from build123d import *

# Parameters (mm, degrees)
BOSS_EXTRUDE1_DEPTH      = 10
BOSS_EXTRUDE1_DEPTH_BACK = 10
SKETCH2_W                = 17.5
SKETCH2_H                = 24
SKETCH3_W                = 9.984775587
SKETCH3_H                = 3
SKETCH3_W_2              = 10
CUT_EXTRUDE1_DEPTH       = 10


with BuildPart() as part:
    # Sketch2 → Boss-Extrude1 (new, two sides: drawn at the far end of the back side and taken through both)
    with BuildSketch(Plane.XY.offset(-BOSS_EXTRUDE1_DEPTH_BACK)):
        with Locations((8.75, -33)):
            Rectangle(SKETCH2_W, SKETCH2_H)
        with Locations((-8.75, -33)):
            Rectangle(SKETCH2_W, SKETCH2_H)
        Polygon((28.106601718, -45), (17.5, -45), (17.5, -21), (24.571067812, -13.928932188), (28.106601718, -17.464466094), align=None)
        Polygon((-28.106601718, -17.464466094), (-28.106601718, -45), (-17.5, -45), (-17.5, -21), (-24.571067812, -13.928932188), align=None)
    extrude(amount=BOSS_EXTRUDE1_DEPTH + BOSS_EXTRUDE1_DEPTH_BACK)

    # Sketch3 → Cut-Extrude1 (cut)
    with BuildSketch(Plane(origin=(0, 0, -10), x_dir=(-1, 0, 0), z_dir=(0, 0, -1))):
        with Locations((-4.992387794, -34.5)):
            Rectangle(SKETCH3_W, SKETCH3_H)
        with Locations((5, -34.5)):
            Rectangle(SKETCH3_W_2, SKETCH3_H)
    extrude(amount=-CUT_EXTRUDE1_DEPTH, mode=Mode.SUBTRACT)


solid = part.part
Work out the finished part from the listing and answer in its coordinate system (mm). A direction names the side the tool comes from. Round coordinates to 2 decimals unless told otherwise and drop trailing zeros. Write each loop counter-clockwise with the first axis right and the second up, starting at its lowest first coordinate (ties: lowest second). Pieces come first, ordered by that corner, then holes.
1) A cutting plane is placed at D-D (z = -8.5). Give the vertices of the cut face in (x, y), plus the area to 3 significant figures.
2) A cutting plane is placed at C-C (y = -34). Give the vertices of the cut face in (x, z), plus the area to 3 significant figures.
3) Straight lines are drawn through the part: line 1 (Y direction, x = 7, z = -4.5); line 2 (Y direction, x = 0, z = 7.25); line 3 (X direction, y = -16, z = -0.5). For each, find the intervals that lie inside material, in ascending order.
4) The mould has two halves that part along Y. Classify faces 4 (the flat face through (0, -33, -5)), 5 (the flat face through (0, -33, 10)), 6 (the flat face through (0, -36, -5)), 7 (the flat face through (-26.31, -15.67, -0.14)): pulls with the +Y half, pulls with the -Y half, needs draft (parallel to the pull), parting line crosses it, or undercut.
5) A cutting plane is placed at B-B (x = -8). Give the vertices of the cut face in (y, z), plus the area to 3 significant figures.
6) Given pin 1 Ø8 at (x, z) = (1.5, -4) entering from +Y, flat-ended and moving along its own axis, determine where the tip first touches the part or whether it passes through.
7) A tool of negligible diameter and unlimited length cuts with its end or side. For faces 1 (the flat face through (9.985, -35, -5)), 2 (the flat face through (21, -17.5, -0.1)), 3 (the flat face through (26.31, -15.67, -0.14)), from which of +Z, -Z, +X, -X, +Y, -Y can it reach the whole face along a straight path? Write none if from no direction.
8) A cutting plane is placed at A-A (y = -20). Give the vertices of the cut face in (x, z), plus the area to 3 significant figures.
Completed:
1. outline: (-28.11, -45) - (28.11, -45) - (28.11, -17.46) - (24.57, -13.93) - (17.5, -21) - (-17.5, -21) - (-24.57, -13.93) - (-28.11, -17.46) - close; hole (-10, -36) - (9.98, -36) - (9.98, -33) - (-10, -33) - close
1. area: 1,380 mm2
2. outline: (-28.11, -10) - (-10, -10) - (-10, 0) - (9.98, 0) - (9.98, -10) - (28.11, -10) - (28.11, 10) - (-28.11, 10) - close
2. area: 924 mm2
3. line 1: y = -45 to -36, -33 to -21
3. line 2: y = -45 to -21
3. line 3: x = -26.64 to -22.5, 22.5 to 26.64
4. face 4: undercut
4. face 5: needs draft
4. face 6: undercut
4. face 7: pulls with the +Y half
5. outline: (-45, -10) - (-36, -10) - (-36, 0) - (-33, 0) - (-33, -10) - (-21, -10) - (-21, 10) - (-45, 10) - close
5. area: 450 mm2
6. pin 1: stops at y = -21
7. face 1: -Z
7. face 2: +Z, -Z, +Y
7. face 3: +Z, -Z, +X, +Y
8. outline: (-28.11, -10) - (-18.5, -10) - (-18.5, 10) - (-28.11, 10) - close; (18.5, -10) - (28.11, -10) - (28.11, 10) - (18.5, 10) - close
8. area: 384 mm2
